The model under review builds one solid part; all positions refer to its coordinate system, in mm. A direction names the side the tool comes from. Coordinates: 2 decimals unless noted, no trailing zeros. Loops run counter-clockwise (first coordinate to the right, second up) from the corner with the lowest first, then second, coordinate; pieces in that order, holes last. Notation, with made-up numbers: M 33,-35 L 62,-35 A34 ccw 62,-4 Z; hole C 73,46 d10. An arc over 180 degrees is marked long. Return JSON: item names as keys, results as strings.
```python
from build123d import *

# Parameters (mm, degrees)
SKETCH1_W           = 16.57424281
SKETCH1_H           = 6
BOSS_EXTRUDE1_DEPTH = 3
SKETCH2_R           = 2.181797835
SKETCH2_R_2         = 1.963463841
BOSS_EXTRUDE2_DEPTH = 6
FILLET2_R           = 1
FILLET3_R           = 0.3


with BuildPart() as part:
    # Sketch1 → Boss-Extrude1 (new body)
    with BuildSketch(Plane.XY):
        Rectangle(SKETCH1_W, SKETCH1_H)
    extrude(amount=BOSS_EXTRUDE1_DEPTH)

    # Sketch2 → Boss-Extrude2 (add)
    # profile 1 of 3: a face of its own
    with BuildSketch(Plane.XY.offset(3)):
        with Locations((-5.454256394, 0)):
            Circle(SKETCH2_R)
        with Locations((-5.454256394, 0)):
            Circle(SKETCH2_R_2, mode=Mode.SUBTRACT)
    # profile 2 of 3: a face of its own
    with BuildSketch(Plane.XY.offset(3)):
        with Locations(Location((5.454256394, 0, 0), (0, 0, 180))):
            Circle(SKETCH2_R)
        with Locations(Location((5.454256394, 0, 0), (0, 0, 180))):
            Circle(SKETCH2_R_2, mode=Mode.SUBTRACT)
    # profile 3 of 3: a face of its own
    with BuildSketch(Plane.XY.offset(3)):
        Polygon((-2.055965806, -2.429777771), (2.055965806, -2.429777771), (2.973504265, 0.356820512), (2.157914524, 1.699145294), (-2.157914524, 1.699145294), (-2.973504265, 0.356820512), align=None)
        Polygon((-1.920034182, -2.242871788), (1.920034182, -2.242871788), (2.803589735, 0.356820512), (2.055965806, 1.529230765), (-2.055965806, 1.529230765), (-2.803589735, 0.356820512), align=None, mode=Mode.SUBTRACT)
    extrude(amount=BOSS_EXTRUDE2_DEPTH)

    # Fillet2
    fillet2_edges = [part.edges().sort_by_distance(p)[0] for p in [
        (8.287121405, -3, 1.5),
        (-8.287121405, -3, 1.5),
        (-8.287121405, 3, 1.5),
        (8.287121405, 3, 1.5),
    ]]
    fillet(fillet2_edges, radius=FILLET2_R)

    # Fillet3
    fillet3_edges = [part.edges().sort_by_distance(p)[0] for p in [
        (-2.157914524, 1.699145294, 6),
        (-2.973504265, 0.356820512, 6),
        (-2.055965806, -2.429777771, 6),
        (2.055965806, -2.429777771, 6),
        (2.973504265, 0.356820512, 6),
        (2.157914524, 1.699145294, 6),
    ]]
    fillet(fillet3_edges, radius=FILLET3_R)


solid = part.part
```
1. Insertion check: pin 1 Ø3 at (x, z) = (0.5, 6) entering from -Y; pin 2 Ø1 at (x, z) = (-2, 4.5) entering from +Y; pin 3 Ø2 at (x, y) = (5.5, 0) entering from +Z. Each pin has a flat end and moves straight along its axis. Give the tip position at first contact, or say it passes through.
Check values:
{"pin 1": "y = -2.43", "pin 2": "y = 1.7", "pin 3": "z = 3"}
2. Add section A-A on z = 3.5. Give the boundary of the cut face in (x, y).
Check values:
{"outline": "C -5.45,0 d4.36; M -2.93,0.23 L -2.12,-2.22 A0.3 ccw -1.84,-2.43 L 1.84,-2.43 A0.3 ccw 2.12,-2.22 L 2.93,0.23 A0.3 ccw 2.9,0.48 L 2.25,1.55 A0.3 ccw 1.99,1.7 L -1.99,1.7 A0.3 ccw -2.25,1.55 L -2.9,0.48 A0.3 ccw Z; C 5.45,0 d4.36; hole C -5.45,0 d3.93; hole M -2.8,0.36 L -1.92,-2.24 L 1.92,-2.24 L 2.8,0.36 L 2.06,1.53 L -2.06,1.53 Z; hole C 5.45,0 d3.93"}
3. Add section B-B on x = 0.5. Give the boundary of the cut face in (y, z), plus the area to 3 significant figures.
Check values:
{"outline": "M -3,0 L 3,0 L 3,3 L 1.7,3 L 1.7,9 L 1.53,9 L 1.53,3 L -2.24,3 L -2.24,9 L -2.43,9 L -2.43,3 L -3,3 Z", "area": "20.1 mm²"}
4. Add section C-C on y = -1.35. Give the boundary of the cut face in (x, z), plus the area to 3 significant figures.
Check values:
{"outline": "M -8.29,0 L 8.29,0 L 8.29,3 L 7.17,3 L 7.17,9 L 6.88,9 L 6.88,3 L 4.03,3 L 4.03,9 L 3.74,9 L 3.74,3 L 2.41,3 L 2.41,9 L 2.22,9 L 2.22,3 L -2.22,3 L -2.22,9 L -2.41,9 L -2.41,3 L -3.74,3 L -3.74,9 L -4.03,9 L -4.03,3 L -6.88,3 L -6.88,9 L -7.17,9 L -7.17,3 L -8.29,3 Z", "area": "58.9 mm²"}
5. To check wall thickness, follow line 1 (Y direction, x = 0.25, z = 4.5); line 2 (Y direction, x = -5.5, z = 6.75); line 3 (Z direction, x = 0.25, y = 0.25). State the ranges of each line that lie inside material, in increasing order.
Check values:
{"line 1": "-2.43 to -2.24, 1.53 to 1.7", "line 2": "-2.18 to -1.96, 1.96 to 2.18", "line 3": "0 to 3"}
6. The part is to be moulded in two halves that separate along Y. For faces 6 (the face through (-5, 0, 3)), 7 (the face through (7.012, 1.195, 5.958)), 8 (the face through (7.634, -0.096, 5.958)), 9 (the face through (2.578, 1.007, 5.958)), say which applies: released by +Y, released by -Y, zero draft, split by the parting line, or undercut.
Check values:
{"face 6": "undercut", "face 7": "undercut", "face 8": "split by the parting line", "face 9": "released by +Y"}
7. Machinability: for faces 1 (the face through (-2.57, 1.02, 5.96)), 2 (the face through (-2.533, -0.982, 5.958)), 3 (the face through (8, -2.7, 1.5)), 4 (the face through (0, 1.529, 6)), 5 (the face through (-8, 2.7, 1.5)), which of the approach directions +Z, -Z, +X, -X, +Y, -Y give a long, thin tool a straight path to every point of the face, cutting with its end or side? Answer none if there is none.
Check values:
{"face 1": "+Z, +Y", "face 2": "+Z, -Y", "face 3": "+Z, -Z, +X, -Y", "face 4": "+Z", "face 5": "+Z, -Z, -X, +Y"}
8. Add section D-D on x = 2.5. Give the boundary of the cut face in (y, z), plus the area to 3 significant figures.
Check values:
{"outline": "M -3,0 L 3,0 L 3,3 L 1.14,3 L 1.14,9 L 0.83,9 L 0.83,3 L -0.54,3 L -0.54,9 L -1.08,9 L -1.08,3 L -3,3 Z", "area": "23.1 mm²"}
